Here's how the part is built. I have some questions about the finished solid (model axes, mm). Face numbers are marked on the shaded views. A direction names the side the tool comes from. Give positions to 0.01 mm unless a question says otherwise; leave off trailing zeros. Write each loop counter-clockwise with the first axis right and the second up, starting at its lowest first coordinate (ties: lowest second). Pieces come first, ordered by that corner, then holes. Notation, with made-up numbers: (17, 42.25) - (31, 42.25) arc R22 cw to (31, 62.25) - close; hole circle Ø6 at (36, 89.5). An arc over 180 degrees is marked (long way). Write each question's results on one line, items separated by ' | '. Start each with the question number.
Item 1: Please list where these lines run through material, in increasing order: line 1 along Z through (x, y) = (0, 58); line 2 along X through (y, z) = (30, -116); line 3 along X through (y, z) = (57, -121.5).
Item 2: Will these pins go through, and if not, where does the flat tip stop? P1, Ø12, axis at x = -69.5, z = 122, coming from the -Y side (3 decimals); P2, Ø5, axis at x = 124, y = 94.5, coming from the +Z side; P3, Ø21, axis at x = 94.5, z = 5.5, coming from the -Y side; P4, Ø8, axis at y = 3.5, z = 58.5, coming from the -X side.
Item 3: Suppose I cut it at B-B on y = 17.5. Count the separate pieces of the cut face and the enclosed holes in it, then the cut area to 3 significant figures.
Item 4: Suppose I cut it at D-D on x = -98. List the corners of the cut face in (y, z) for me (3 decimals), then the cut area to 3 significant figures.
Item 5: We'd pull the mould along Z, two halves only. Please class the marked faces 4, 5, 6 and 7: +Z half, -Z half, draft (parallel to the pull), parting line (faces both ways), or undercut.
Item 6: Suppose I cut it at A-A on x = 0. List the corners of the cut face in (y, z) for me, then the cut area to 3 significant figures.
Item 7: Which directions (+Z, -Z, +X, -X, +Y, -Y) give clear straight access to the entire face, cutting with the end or side of a thin tool? Please do the marked faces 1, 2 and 3.
Autodesk Inventor part; units mm, degrees
ref_plane "YZ Plane" through (0, 0, 0) normal (1, 0, 0) x (0, 1, 0)
ref_plane "XZ Plane" through (0, 0, 0) normal (0, 1, 0) x (-1, 0, 0)
ref_plane "XY Plane" through (0, 0, 0) normal (0, 0, 1) x (1, 0, 0)
sketch "Sketch1" plane through (0, 0, 0) normal (0, 1, 0) x (-1, 0, 0)
  circle A0 centre (0, 0) radius 139.7
  circle A1 centre (0, 0) radius 138.1125
  dimension "d0" = 279.4
  dimension "d1" = 276.225
extrude "Extrusion1" add sketch "Sketch1" along normal blind 101.6
sketch "Sketch2" plane through (0, 101.6, 0) normal (0, 1, 0) x (1, 0, 0)
  line L0 (88.9, 14.2875) -> (247.65, 14.2875)
  line L1 (247.65, 14.2875) -> (247.65, -14.2875)
  line L2 (247.65, -14.2875) -> (88.9, -14.2875)
  line L3 (88.9, -14.2875) -> (88.9, 14.2875)
  line L4 (88.9, 14.2875) -> (247.65, -14.2875) construction
  line L5 (247.65, 14.2875) -> (88.9, -14.2875) construction
  circle A0 centre (0, 0) radius 139.7
  point P0 (168.275, 0)
  point P1 (168.275, 0)
  point P2 (139.7, 0)
  dimension "d4" = 158.75
  dimension "d5" = 28.575
  dimension "d7" = 107.95
extrude "Extrusion2" add sketch "Sketch2" along normal blind 28.575 contours L0 A0 L2 L3 | L0 L1 L2 A0 picked at (105.8333, 0)
sketch "Sketch3" plane through (0, 101.6, 0) normal (0, -1, 0) x (1, 0, 0)
  line L0 (247.65, -14.2875) -> (88.9, -14.2875)
  line L1 (107.95, 14.2875) -> (136.525, 14.2875)
  line L2 (136.525, 14.2875) -> (136.525, -14.2875)
  line L3 (136.525, -14.2875) -> (107.95, -14.2875)
  line L4 (107.95, -14.2875) -> (107.95, 14.2875)
  line L5 (107.95, 14.2875) -> (136.525, -14.2875) construction
  line L6 (136.525, 14.2875) -> (107.95, -14.2875) construction
  line L7 (88.9, 14.2875) -> (88.9, -14.2875)
  line L8 (137.3715, 14.2875) -> (88.9, 14.2875)
  point P0 (0, 0)
  point P1 (122.2375, 0)
  dimension "d10" = 28.575
  dimension "d11" = 19.05
extrude "Extrusion3" add sketch "Sketch3" along normal blind 149.225 contours L0 L4 L1 L2
pattern_circular "Circular Pattern1" count 3 over 360 about axis through (0, 0, 0) along (0, 1, 0) of "Extrusion2", "Extrusion3"
properties part number "Burner-Placeholder"
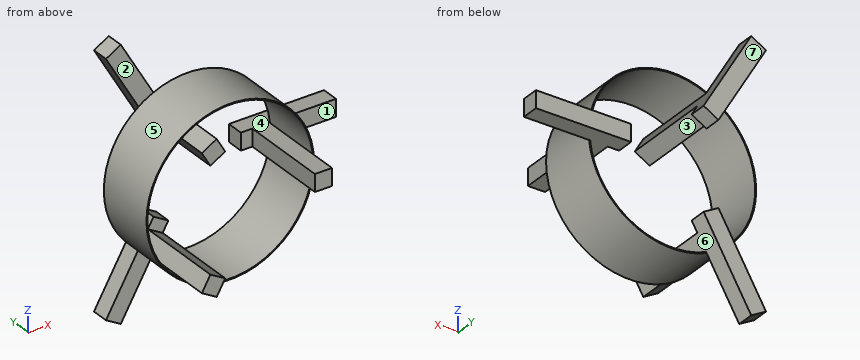
Checked values:
1) line 1: z = -139.7 to -138.11, 138.11 to 139.7 | line 2: x = -77.85 to -74.96, -72.13 to -50.47, 74.96 to 77.85 | line 3: x = -68.95 to -65.67, -62.61 to -53.65, 65.67 to 68.95
2) P1: stops at y = -47.625 | P2: stops at z = 68.95 | P3: stops at y = 101.6 | P4: stops at x = -128.63
3) separate pieces: 4 | enclosed holes: 1 | area: 3,840 mm^2
4) outline: (0, -99.559) - (101.6, -99.559) - (101.6, -97.319) - (0, -97.319) - close; (0, 97.319) - (101.6, 97.319) - (101.6, 99.559) - (0, 99.559) - close; (101.6, -198.316) - (130.175, -198.316) - (130.175, -141.166) - (101.6, -141.166) - close; (101.6, 141.166) - (130.175, 141.166) - (130.175, 198.316) - (101.6, 198.316) - close | area: 3,720 mm^2
5) face 4: undercut | face 5: parting line | face 6: undercut | face 7: draft
6) outline: (0, -139.7) - (101.6, -139.7) - (101.6, -138.11) - (0, -138.11) - close; (0, 138.11) - (101.6, 138.11) - (101.6, 139.7) - (0, 139.7) - close | area: 323 mm^2
7) face 1: +Z, -Z, +X, -Y | face 2: +Z, -X, -Y | face 3: -Y
